Design review of the part built by this model. Coordinates are the model's own, in mm. A direction names the side the tool comes from. Coordinates: 2 decimals unless noted, no trailing zeros. Loops run counter-clockwise (first coordinate to the right, second up) from the corner with the lowest first, then second, coordinate; pieces in that order, holes last. Notation, with made-up numbers: (-23, 12.5) -> (0, 12.5) arc R37 cw to (0, 50.5) -> close; hole circle Ø7 at (11, -15.75). An arc over 180 degrees is marked (long way). Answer as a JSON object with one key per item and string values.
```python
from build123d import *

# Parameters (mm, degrees)
F0_W     = 50.8
F0_H     = 101.6
F1_DEPTH = 25.4
F2_W     = 50.8
F2_H     = 12.7
F3_DEPTH = 6.35
F4_W     = 50.8
F4_H     = 12.7
F5_DEPTH = 6.35


with BuildPart() as f1:
    # F0 (on Front) → F1 (new body)
    with BuildSketch(Plane.XZ):
        Rectangle(F0_W, F0_H)
    extrude(amount=F1_DEPTH)

    # F2 (on face) → F3 (join)
    with BuildSketch(Plane.XZ.offset(25.4)):
        Rectangle(F2_W, F2_H)
    extrude(amount=F3_DEPTH)

    # F4 (on face) → F5 (join)
    with BuildSketch(Plane.XZ.offset(25.4)):
        with Locations((0, 22.225)):
            Rectangle(F4_W, F4_H)
        with Locations((0, 40.902834)):
            Rectangle(F4_W, F4_H)
        with Locations((0, -21.466311)):
            Rectangle(F4_W, F4_H)
        with Locations((0, -41.953252)):
            Rectangle(F4_W, F4_H)
    extrude(amount=F5_DEPTH)


solid = f1.part
```
1) Add section A-A, the plane y = -28. Give the boundary of the cut face in (x, z) (3 decimals).
Completed:
{"outline": "(-25.4, -48.303) -> (25.4, -48.303) -> (25.4, -35.603) -> (-25.4, -35.603) -> close; (-25.4, -27.816) -> (25.4, -27.816) -> (25.4, -15.116) -> (-25.4, -15.116) -> close; (-25.4, -6.35) -> (25.4, -6.35) -> (25.4, 6.35) -> (-25.4, 6.35) -> close; (-25.4, 15.875) -> (25.4, 15.875) -> (25.4, 28.575) -> (-25.4, 28.575) -> close; (-25.4, 34.553) -> (25.4, 34.553) -> (25.4, 47.253) -> (-25.4, 47.253) -> close"}
2) Add section B-B, the plane x = -11. Give the boundary of the cut face in (y, z) (3 decimals).
Completed:
{"outline": "(-31.75, -48.303) -> (-25.4, -48.303) -> (-25.4, -50.8) -> (0, -50.8) -> (0, 50.8) -> (-25.4, 50.8) -> (-25.4, 47.253) -> (-31.75, 47.253) -> (-31.75, 34.553) -> (-25.4, 34.553) -> (-25.4, 28.575) -> (-31.75, 28.575) -> (-31.75, 15.875) -> (-25.4, 15.875) -> (-25.4, 6.35) -> (-31.75, 6.35) -> (-31.75, -6.35) -> (-25.4, -6.35) -> (-25.4, -15.116) -> (-31.75, -15.116) -> (-31.75, -27.816) -> (-25.4, -27.816) -> (-25.4, -35.603) -> (-31.75, -35.603) -> close"}
3) Clearance check with flat-ended pins moving along their axes: pin 1 Ø6.5 at (x, z) = (10.5, 30.5) entering from -Y; pin 2 Ø7 at (x, y) = (-12, -29) entering from +Z; pin 3 Ø4 at (x, z) = (5.5, -8.5) entering from -Y; pin 4 Ø5 at (x, y) = (11, -28.5) entering from -Z. State where each tip first meets the part, or that it passes through.
Completed:
{"pin 1": "y = -31.75", "pin 2": "z = 47.25", "pin 3": "y = -25.4", "pin 4": "z = -48.3"}
4) The part is to be moulded in two halves that separate along Z. For faces 1 (the flat face through (0, -29, -6.35)), 2 (the flat face through (0, -29, 47.253)), 3 (the flat face through (0, 0, 1)), 4 (the flat face through (0, -29, -48.303)), say which applies: pulls with the +Z half, pulls with the -Z half, needs draft (parallel to the pull), parting line crosses it, or undercut.
Completed:
{"face 1": "undercut", "face 2": "pulls with the +Z half", "face 3": "needs draft", "face 4": "pulls with the -Z half"}
5) For faces 5 (the flat face through (0, -29, 6.35)), 6 (the flat face through (0, -31.75, -42)), 7 (the flat face through (0, -25.4, -50)), list the 3-axis set-ups (+Z, -Z, +X, -X, +Y, -Y) from which the entire face can be reached by the end or side of a thin tool; tool diameter is ignored.
Completed:
{"face 5": "+X, -X, -Y", "face 6": "+Z, -Z, +X, -X, -Y", "face 7": "-Z, +X, -X, -Y"}
6) Add section C-C, the plane z = 8. Give the boundary of the cut face in (x, y), and give its area (3 significant figures).
Completed:
{"outline": "(-25.4, -25.4) -> (25.4, -25.4) -> (25.4, 0) -> (-25.4, 0) -> close", "area": "1,290 mm²"}
7) Wall thickness on probe 1 along Z at (x, y) = (-7.5, -29) (3 decimals); probe 2 along Y at (x, z) = (-17.5, -31): over which ranges is each line inside the solid? List them lowest first.
Completed:
{"probe 1": "-48.303 to -35.603, -27.816 to -15.116, -6.35 to 6.35, 15.875 to 28.575, 34.553 to 47.253", "probe 2": "-25.4 to 0"}
